from build123d import *

# Parameters (mm, degrees)
PAD047_DEPTH    = 42
SKETCH076_R     = 18
SKETCH076_R_2   = 1.5
POCKET023_DEPTH = 2
PAD048_DEPTH    = 1.5
PAD049_DEPTH    = 1.4
SKETCH079_W     = 8
SKETCH079_H     = 2
PAD050_DEPTH    = 32
SKETCH080_W     = 8
SKETCH080_H     = 2
PAD051_DEPTH    = 32
SKETCH081_W     = 1.5
SKETCH081_H     = 42
PAD052_DEPTH    = 17
SKETCH082_R     = 1.75
POCKET024_DEPTH = 5
FILLET002_R     = 5


with BuildPart() as part:
    # Sketch075 → Pad047 (new body)
    with BuildSketch(Plane.XZ):
        Polygon((-21, 0), (21, 0), (21, 1.5), (0, 35), (0, 32.17586), (19.229644, 1.5), (-19.5, 1.5), (-19.5, 35), (-21, 35), align=None)
    extrude(amount=PAD047_DEPTH)

    # Sketch076 (on Face2 of Pad047) → Pocket023 (cut)
    with BuildSketch(Plane(origin=(0, 0, 0), x_dir=(1, 0, 0), z_dir=(0, 0, -1))):
        with Locations((0, 21)):
            Circle(SKETCH076_R)
        with Locations((-16, 37)):
            Circle(SKETCH076_R_2)
        with Locations((16, 37)):
            Circle(SKETCH076_R_2)
        with Locations((16, 5)):
            Circle(SKETCH076_R_2)
        with Locations((-16, 5)):
            Circle(SKETCH076_R_2)
    extrude(amount=-POCKET023_DEPTH, mode=Mode.SUBTRACT)

    # Sketch077 (on Face4 of Pocket023) → Pad048 (join)
    with BuildSketch(Plane(origin=(0, 0, 0), x_dir=(1, 0, 0), z_dir=(0, 1, 0))):
        Polygon((-21, -35), (0, -35), (21, -1.5), (21, 0), (-21, 0), align=None)
    extrude(amount=PAD048_DEPTH)

    # Sketch078 (on Face1 of Pad048) → Pad049 (join)
    with BuildSketch(Plane.XZ.offset(42)):
        Polygon((-21, 35), (-21, 0), (21, 0), (21, 1.5), (0, 35), align=None)
    extrude(amount=PAD049_DEPTH)

    # Sketch079 (on Face14 of Pad049) → Pad050 (join)
    with BuildSketch(Plane(origin=(0, 1.5, 0), x_dir=(1, 0, 0), z_dir=(0, 1, 0))):
        with Locations((-17, -1)):
            Rectangle(SKETCH079_W, SKETCH079_H)
    extrude(amount=PAD050_DEPTH)

    # Sketch080 (on Face1 of Pad050) → Pad051 (join)
    with BuildSketch(Plane.XZ.offset(43.4)):
        with Locations((-17, 1)):
            Rectangle(SKETCH080_W, SKETCH080_H)
    extrude(amount=PAD051_DEPTH)

    # Sketch081 (on Face1 of Pad051) → Pad052 (join)
    with BuildSketch(Plane.XZ.offset(43.4)):
        with Locations((0.75, 21)):
            Rectangle(SKETCH081_W, SKETCH081_H)
    extrude(amount=PAD052_DEPTH)

    # Sketch082 (on Face5 of Pad052) → Pocket024 (cut)
    with BuildSketch(Plane(origin=(0, 0, 0), x_dir=(0, 0, -1), z_dir=(-1, 0, 0))):
        with Locations((-39, 51.9)):
            Circle(SKETCH082_R)
        with Locations((-3, 51.9)):
            Circle(SKETCH082_R)
        with BuildLine():
            ThreePointArc((-28, 57.9), (-34, 51.9), (-28, 45.9))
            Line((-28, 45.9), (-14, 45.9))
            ThreePointArc((-14, 45.9), (-8, 51.9), (-14, 57.9))
            Line((-28, 57.9), (-14, 57.9))
        make_face()
    extrude(amount=-POCKET024_DEPTH, mode=Mode.SUBTRACT)

    # Fillet002
    fillet002_edges = [part.edges().sort_by_distance(p)[0] for p in [
        (0.75, -43.4, 42),
        (0.75, -60.4, 42),
        (0.75, -60.4, 0),
        (-13, -43.4, 1),
        (-13, 1.5, 1),
    ]]
    fillet(fillet002_edges, radius=FILLET002_R)


solid = part.part
Design review of the part built by this model. Coordinates are the model's own, in mm. A direction names the side the tool comes from. Give positions to 0.01 mm unless a question says otherwise; leave off trailing zeros. Order: outer loops, then holes, each group sorted by start corner. A loop starts at its lowest first (then second) coordinate and runs counter-clockwise, first axis right, second up.
1. To check wall thickness, follow L1, parallel to Z at x = 0.9, y = -51.9; L2, parallel to Y at x = -1, z = 10; L3, parallel to X at y = -37, z = 1. State the ranges of each line that lie inside material, in increasing order.
Solution:
L1: z = 0 to 1.25, 4.75 to 8, 34 to 37.25, 40.75 to 42
L2: y = -43.4 to -42, 0 to 1.5
L3: x = -21 to -17.5, -14.5 to -8.25, 8.25 to 14.5, 17.5 to 21
2. Mouldability with a two-part tool opening along X and no side actions: class faces 1 (the flat face through (9.48, -20.71, 17.05)), 2 (the flat face through (-13, 20, 1)), 3 (the flat face through (-21, -20, 13)) as +X half, -X half, draft (parallel to the pull), parting line (faces both ways), or undercut.
Solution:
face 1: undercut
face 2: +X half
face 3: -X half
3. Add section B-B, the plane z = 22. State the section outline as (x, y) points, then the cut area to 3 significant figures.
Solution:
outline: (-21, -43.4) - (0, -43.4) - (0, -45.9) - (1.5, -45.9) - (1.5, -43.4) - (8.15, -43.4) - (8.15, 1.5) - (-21, 1.5) - close; (0, -60.4) - (1.5, -60.4) - (1.5, -57.9) - (0, -57.9) - close; hole (-19.5, -42) - (6.38, -42) - (6.38, 0) - (-19.5, 0) - close
area: 229 mm2
4. Add section A-A, the plane y = -51.9. State the section outline as (x, z) points.
Solution:
outline: (-21, 0) - (-13, 0) - (-13, 2) - (-21, 2) - close; (0, 0) - (1.5, 0) - (1.5, 1.25) - (0, 1.25) - close; (0, 4.75) - (1.5, 4.75) - (1.5, 8) - (0, 8) - close; (0, 34) - (1.5, 34) - (1.5, 37.25) - (0, 37.25) - close; (0, 40.75) - (1.5, 40.75) - (1.5, 42) - (0, 42) - close
5. For pin 1 Ø2 at (y, z) = (23.5, 1) entering from +X; pin 2 Ø12 at (x, y) = (-15, -14) entering from +Z; pin 3 Ø1.2 at (x, z) = (1, 22.5) entering from +Y, all flat-tipped, find the tip position at first contact; note any pin that passes through.
Solution:
pin 1: stops at x = -13
pin 2: stops at z = 35
pin 3: stops at y = 1.5
6. Add section C-C, the plane x = -16. State the section outline as (y, z) points, then the cut area to 3 significant figures.
Solution:
outline: (-75.4, 0) - (-38.5, 0) - (-38.5, 1.5) - (-42, 1.5) - (-42, 35) - (-43.4, 35) - (-43.4, 2) - (-75.4, 2) - close; (-35.5, 0) - (-29.25, 0) - (-29.25, 1.5) - (-35.5, 1.5) - close; (-12.75, 0) - (-6.5, 0) - (-6.5, 1.5) - (-12.75, 1.5) - close; (-3.5, 0) - (33.5, 0) - (33.5, 2) - (1.5, 2) - (1.5, 35) - (0, 35) - (0, 1.5) - (-3.5, 1.5) - close
area: 259 mm2
7. Add section D-D, the plane y = -1.5. State the section outline as (x, z) points.
Solution:
outline: (-21, 0) - (21, 0) - (21, 1.5) - (0, 35) - (0, 32.18) - (19.23, 1.5) - (-19.5, 1.5) - (-19.5, 35) - (-21, 35) - close
8. Tool access review of faces 4 (the flat face through (-5, 0, 18)), 5 (the flat face through (-16, 17, 2)), 6 (the cylindrical face through (14.5, -5.07, 0.74)), 7 (the flat face through (9, -43.4, 13)): name each direction out of +Z, -Z, +X, -X, +Y, -Y from which nothing blocks a thin tool from reaching the whole face with its end or side.
Solution:
face 4: none
face 5: +Z, +X, -X, +Y
face 6: -Z
face 7: +Z, -Z, +X, -Y
